Build history of the part. All positions in model axes, mm. Face numbers are marked on the shaded views. Give positions to 0.01 mm unless a question says otherwise; leave off trailing zeros. Order: outer loops, then holes, each group sorted by start corner. A loop starts at its lowest first (then second) coordinate and runs counter-clockwise, first axis right, second up. Notation, with made-up numbers: M 5,25.5 L 45,25.5 A5 cw 45,32.5 Z; hole C 85.5,22.5 d11. An arc over 180 degrees is marked long. One line per item, written item: value.
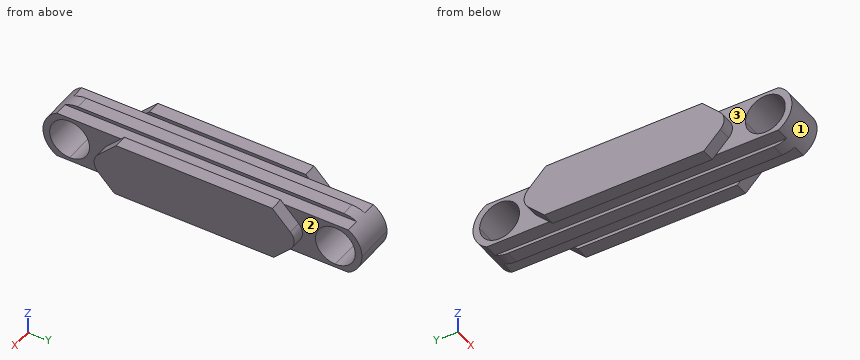
from build123d import *

# Parameters (mm, degrees)
F1_DEPTH = 45.72
F3_DEPTH = 76.2
F2_W     = 30.48
F2_H     = 7.62
F4_DEPTH = 762
F5_R     = 30.48


with BuildPart() as f1:
    # F0 (on Right) → F1 (new body, symmetric)
    with BuildSketch(Plane.YZ):
        with BuildLine():
            ThreePointArc((0, 45.72), (32.3289220358, 32.3289220358), (45.72, 0))
            ThreePointArc((45.72, 0), (32.3289220358, -32.3289220358), (0, -45.72))
            Line((0, -45.72), (0, -60.96))
            ThreePointArc((0, -60.96), (43.1052293811, -43.1052293811), (60.96, 0))
            ThreePointArc((60.96, 0), (43.1052293811, 43.1052293811), (0, 60.96))
            Line((0, 60.96), (0, 45.72))
        make_face()
        with BuildLine():
            ThreePointArc((0, -45.72), (-45.72, 0), (0, 45.72))
            Line((0, 45.72), (0, 60.96))
            ThreePointArc((0, 60.96), (-43.1052293811, 43.1052293811), (-60.96, 0))
            ThreePointArc((-60.96, 0), (-60.9300804884, -1.9096836578), (-60.8403513231, -3.8174927486))
            ThreePointArc((-60.8403513231, -3.8174927486), (-41.7337228272, -44.434423356), (0, -60.96))
            Line((0, -60.96), (0, -45.72))
        make_face()
        with BuildLine():
            ThreePointArc((-60.96, 0), (-43.1052293811, 43.1052293811), (0, 60.96))
            Line((0, 60.96), (-60.96, 60.96))
            Line((-60.96, 60.96), (-60.96, 0))
        make_face()
        with BuildLine():
            Line((-121.92, -60.96), (0, -60.96))
            ThreePointArc((0, -60.96), (-41.7337228272, -44.434423356), (-60.8403513231, -3.8174927486))
            Line((-60.8403513231, -3.8174927486), (-62.8089220358, -1.8489220358))
            Line((-62.8089220358, -1.8489220358), (-121.92, -60.96))
        make_face()
        Polygon((-62.8089220358, -1.8489220358), (-60.96, 0), (-60.96, 60.96), (-125.6178440717, 60.96), align=None)
        Polygon((-304.8, -60.96), (-121.92, -60.96), (-62.8089220358, -1.8489220358), (-125.6178440717, 60.96), (-304.8, 60.96), align=None)
        Polygon((-487.68, -60.96), (-304.8, -60.96), (-304.8, 60.96), (-483.9821559283, 60.96), (-546.7910779642, -1.8489220358), align=None)
        Polygon((-548.64, -60.96), (-487.68, -60.96), (-546.7910779642, -1.8489220358), (-548.64, -3.6978440717), align=None)
        with BuildLine():
            Line((-546.7910779642, -1.8489220358), (-483.9821559283, 60.96))
            Line((-483.9821559283, 60.96), (-609.6, 60.96))
            ThreePointArc((-609.6, 60.96), (-566.4947706189, 43.1052293811), (-548.64, 0))
            Line((-548.64, 0), (-546.7910779642, -1.8489220358))
        make_face()
        with BuildLine():
            Line((-609.6, -60.96), (-548.64, -60.96))
            Line((-548.64, -60.96), (-548.64, -3.6978440717))
            Line((-548.64, -3.6978440717), (-548.7596486769, -3.8174927486))
            ThreePointArc((-548.7596486769, -3.8174927486), (-567.8662771728, -44.434423356), (-609.6, -60.96))
        make_face()
        with BuildLine():
            ThreePointArc((-548.64, 0), (-566.4947706189, 43.1052293811), (-609.6, 60.96))
            Line((-609.6, 60.96), (-609.6, 45.72))
            ThreePointArc((-609.6, 45.72), (-577.2710779642, 32.3289220358), (-563.88, 0))
            ThreePointArc((-563.88, 0), (-577.2710779642, -32.3289220358), (-609.6, -45.72))
            Line((-609.6, -45.72), (-609.6, -60.96))
            ThreePointArc((-609.6, -60.96), (-567.8662771728, -44.434423356), (-548.7596486769, -3.8174927486))
            ThreePointArc((-548.7596486769, -3.8174927486), (-548.6699195116, -1.9096836578), (-548.64, 0))
        make_face()
        with BuildLine():
            Line((-609.6, 45.72), (-609.6, 60.96))
            ThreePointArc((-609.6, 60.96), (-670.56, 0), (-609.6, -60.96))
            Line((-609.6, -60.96), (-609.6, -45.72))
            ThreePointArc((-609.6, -45.72), (-655.32, 0), (-609.6, 45.72))
        make_face()
        Polygon((-548.64, -3.6978440717), (-546.7910779642, -1.8489220358), (-548.64, 0), align=None)
        with BuildLine():
            ThreePointArc((-60.8403513231, -3.8174927486), (-60.9300804884, -1.9096836578), (-60.96, 0))
            Line((-60.96, 0), (-62.8089220358, -1.8489220358))
            Line((-62.8089220358, -1.8489220358), (-60.8403513231, -3.8174927486))
        make_face()
    extrude(amount=F1_DEPTH, both=True)

    # F0 (on Right) → F3 (join, symmetric)
    with BuildSketch(Plane.YZ):
        Polygon((-487.68, -60.96), (-304.8, -60.96), (-304.8, 60.96), (-483.9821559283, 60.96), (-546.7910779642, -1.8489220358), align=None)
        Polygon((-304.8, -60.96), (-121.92, -60.96), (-62.8089220358, -1.8489220358), (-125.6178440717, 60.96), (-304.8, 60.96), align=None)
    extrude(amount=F3_DEPTH, both=True)

    # F2 (on Front) → F4 (cut, symmetric)
    with BuildSketch(Plane.XZ):
        with Locations((-30.48, 57.15)):
            Rectangle(F2_W, F2_H)
        with Locations((30.48, 57.15)):
            Rectangle(F2_W, F2_H)
        with Locations((-30.48, -57.15)):
            Rectangle(F2_W, F2_H)
        with Locations((30.48, -57.15)):
            Rectangle(F2_W, F2_H)
    extrude(amount=F4_DEPTH, both=True, mode=Mode.SUBTRACT)

    # F5
    f5_edges = [f1.edges().sort_by_distance(p)[0] for p in [
        (60.96, -546.791078, -1.848922),
        (-60.96, -546.791078, -1.848922),
        (-60.96, -62.808922, -1.848922),
        (60.96, -62.808922, -1.848922),
    ]]
    fillet(f5_edges, radius=F5_R)


solid = f1.part
1) Saw through at A-A, the plane y = -18.5. Write the cut outline in (x, z), then the cut area to 3 significant figures.
Check values:
outline: M -45.72,-53.34 L -15.24,-53.34 L -15.24,-60.96 L 15.24,-60.96 L 15.24,-53.34 L 45.72,-53.34 L 45.72,-41.81 L -45.72,-41.81 Z; M -45.72,41.81 L 45.72,41.81 L 45.72,53.34 L 15.24,53.34 L 15.24,60.96 L -15.24,60.96 L -15.24,53.34 L -45.72,53.34 Z
area: 2,570 mm^2
2) Drill centre lines: probe 1 along X at (y, z) = (-446, -54.5); probe 2 along Z at (x, y) = (24, -609.6); probe 3 along Y at (x, z) = (-26.5, -7.5). Where is each one in solid material? Low to high. Write a range as from..to.
Check values:
probe 1: -76.2..-45.72, -15.24..15.24, 45.72..76.2
probe 2: -53.34..-45.72, 45.72..53.34
probe 3: -670.1..-654.7, -564.5..-45.1, 45.1..60.5
3) Mould opens along X. For the marked faces 1, 2 and 3 say: released by +X, released by -X, zero draft, split by the parting line, or undercut.
Check values:
face 1: zero draft
face 2: released by +X
face 3: released by -X
4) Saw through at D-D, the plane y = -241. Write the cut outline in (x, z).
Check values:
outline: M -76.2,-60.96 L -45.72,-60.96 L -45.72,-53.34 L -15.24,-53.34 L -15.24,-60.96 L 15.24,-60.96 L 15.24,-53.34 L 45.72,-53.34 L 45.72,-60.96 L 76.2,-60.96 L 76.2,60.96 L 45.72,60.96 L 45.72,53.34 L 15.24,53.34 L 15.24,60.96 L -15.24,60.96 L -15.24,53.34 L -45.72,53.34 L -45.72,60.96 L -76.2,60.96 Z
5) Saw through at C-C, the plane x = -25.5. Write the cut outline in (y, z).
Check values:
outline: M -639.11,-53.34 L 29.51,-53.34 A60.96 ccw 29.51,53.34 L -639.11,53.34 A60.96 ccw Z; hole C -609.6,0 d91.44; hole M -548.76,-3.82 L -548.64,-3.7 L -548.64,0 A60.96 cw Z; hole C 0,0 d91.44
6) Pin check, flat tips, straight feed: pin 1 (10 mm diameter, centred on x = -56, z = 17.5, fed in from -Y); pin 2 (9 mm diameter, centred on x = 24.5, y = -239, fed in from -Z); pin 3 (1 mm diameter, centred on y = -567, z = 11.5, fed in from +X); pin 4 (10 mm diameter, centred on x = 38.5, z = 26, fed in from -Y). Stop position of each tip, or through.
Check values:
pin 1: y = -530.58
pin 2: z = -53.34
pin 3: through
pin 4: y = -666.83
7) Saw through at B-B, the plane z = 31. Write the cut outline in (x, y).
Check values:
outline: M -76.2,-513.94 L -45.72,-513.94 L -45.72,-575.99 L 45.72,-575.99 L 45.72,-513.94 L 76.2,-513.94 L 76.2,-95.66 L 45.72,-95.66 L 45.72,-33.61 L -45.72,-33.61 L -45.72,-95.66 L -76.2,-95.66 Z; M -45.72,-662.09 L 45.72,-662.09 L 45.72,-643.21 L -45.72,-643.21 Z; M -45.72,33.61 L 45.72,33.61 L 45.72,52.49 L -45.72,52.49 Z
